Here's how the part is built. I have some questions about the finished solid (model axes, mm). A direction names the side the tool comes from. Round coordinates to 2 decimals unless told otherwise and drop trailing zeros. Write each loop counter-clockwise with the first axis right and the second up, starting at its lowest first coordinate (ties: lowest second). Pieces come first, ordered by that corner, then holes. Notation, with made-up numbers: (65.5, -12.75) - (123.5, -12.75) arc R9 cw to (123.5, -6.75) - close; hole circle Ø1 at (16, -28.5). An arc over 180 degrees is marked (long way). One line per item, written item: value. Start each with the question number.
Item 1: Imagine slicing it at D-D, the plane z = -1.5. Please give me the cut outline in (x, y), then the cut area to 3 significant figures.
Item 2: Imagine slicing it at C-C, the plane y = -17. Please give me the cut outline in (x, z).
Item 3: If I drill on line 1 (Y direction, x = 0, z = 2.5); line 2 (X direction, y = 3, z = -8.5), over which ranges is the centre line in solid material (lowest first)?
Item 4: Imagine slicing it at A-A, the plane x = 0. Please give me the cut outline in (y, z).
Item 5: Thinking about a two-plate mould opening in X: for faces 1 (the face through (12.5, 0, 7)), 2 (the face through (-12.5, 0, 7)), 3 (the face through (0, 0, 0)), 4 (the face through (-2.4, 29.5, -19)), which applies, released by +X, released by -X, zero draft, split by the parting line, or undercut?
Item 6: For P1, Ø5, axis at y = -2.5, z = 5, coming from the +X side; P2, Ø8, axis at x = 5, z = 8.5, coming from the +Y side; P3, Ø4, axis at x = 0, y = -7.3, coming from the +Z side; P4, Ø17.5, axis at x = 6, y = -9.5, coming from the -Z side, each with a flat end and sliding along its axis, tell me the tip position at first contact or that it passes through.
Item 7: Imagine slicing it at B-B, the plane x = 7.3. Please give me the cut outline in (y, z).
Item 8: For faces 5 (the face through (30.75, 0, -8)), 6 (the face through (0, -12.5, 7)), 7 (the face through (0, -28.95, -9)), 8 (the face through (0, 12.5, 7)), which set-ups out of +Z, -Z, +X, -X, +Y, -Y let a thin tool reach every point of the face, with its end or its side?
```python
from build123d import *

# Parameters (mm, degrees)
SKETCH_W      = 61.5
SKETCH_H      = 61.5
PAD_DEPTH     = 2
SKETCH001_W   = 61.5
SKETCH001_H   = 61.5
SKETCH001_W_2 = 57.9
SKETCH001_H_2 = 57.9
PAD001_DEPTH  = 19
SKETCH002_W   = 25
SKETCH002_H   = 25
PAD002_DEPTH  = 10
SKETCH003_R   = 2.2
POCKET_DEPTH  = 31.001


with BuildPart() as part:
    # Sketch → Pad (new body)
    with BuildSketch(Plane.XY):
        Rectangle(SKETCH_W, SKETCH_H)
    extrude(amount=PAD_DEPTH)

    # Sketch001 → Pad001 (new body)
    with BuildSketch(Plane(origin=(0, 0, 0), x_dir=(1, 0, 0), z_dir=(0, 0, -1))):
        Rectangle(SKETCH001_W, SKETCH001_H)
        Rectangle(SKETCH001_W_2, SKETCH001_H_2, mode=Mode.SUBTRACT)
    extrude(amount=PAD001_DEPTH)

    # Sketch002 → Pad002 (new body)
    with BuildSketch(Plane.XY.offset(2)):
        Rectangle(SKETCH002_W, SKETCH002_H)
    extrude(amount=PAD002_DEPTH)

    # Sketch003 → Pocket (cut, through all)
    with BuildSketch(Plane.XY.offset(12)):
        with Locations((-7.3, 0)):
            Circle(SKETCH003_R)
        with Locations((7.3, 0)):
            Circle(SKETCH003_R)
        with Locations((0, 7.3)):
            Circle(SKETCH003_R)
        with Locations((0, -7.3)):
            Circle(SKETCH003_R)
    extrude(amount=-POCKET_DEPTH, mode=Mode.SUBTRACT)


solid = part.part
```
Values follow:
1. outline: (-30.75, -30.75) - (30.75, -30.75) - (30.75, 30.75) - (-30.75, 30.75) - close; hole (-28.95, -28.95) - (28.95, -28.95) - (28.95, 28.95) - (-28.95, 28.95) - close
1. area: 430 mm^2
2. outline: (-30.75, -19) - (-28.95, -19) - (-28.95, 0) - (28.95, 0) - (28.95, -19) - (30.75, -19) - (30.75, 2) - (-30.75, 2) - close
3. line 1: y = -12.5 to -9.5, -5.1 to 5.1, 9.5 to 12.5
3. line 2: x = -30.75 to -28.95, 28.95 to 30.75
4. outline: (-30.75, -19) - (-28.95, -19) - (-28.95, 0) - (-9.5, 0) - (-9.5, 12) - (-12.5, 12) - (-12.5, 2) - (-30.75, 2) - close; (-5.1, 0) - (5.1, 0) - (5.1, 12) - (-5.1, 12) - close; (9.5, 0) - (28.95, 0) - (28.95, -19) - (30.75, -19) - (30.75, 2) - (12.5, 2) - (12.5, 12) - (9.5, 12) - close
5. face 1: released by +X
5. face 2: released by -X
5. face 3: undercut
5. face 4: zero draft
6. P1: stops at x = 12.5
6. P2: stops at y = 12.5
6. P3: passes through
6. P4: stops at z = 0
7. outline: (-30.75, -19) - (-28.95, -19) - (-28.95, 0) - (-2.2, 0) - (-2.2, 12) - (-12.5, 12) - (-12.5, 2) - (-30.75, 2) - close; (2.2, 0) - (28.95, 0) - (28.95, -19) - (30.75, -19) - (30.75, 2) - (12.5, 2) - (12.5, 12) - (2.2, 12) - close
8. face 5: +Z, -Z, +X, +Y, -Y
8. face 6: +Z, +X, -X, -Y
8. face 7: -Z
8. face 8: +Z, +X, -X, +Y
